Part model, mm, in its own coordinate system. Face numbers are marked on the shaded views. A direction names the side the tool comes from. Give positions to 0.01 mm unless a question says otherwise; leave off trailing zeros. Order: outer loops, then holes, each group sorted by start corner. A loop starts at its lowest first (then second) coordinate and runs counter-clockwise, first axis right, second up. Notation, with made-up numbers: (19, 33.5) - (46, 33.5) arc R17 ccw to (46, 40.5) - close; hole circle Ø3 at (62.5, 20.5). An arc over 180 degrees is marked (long way). One line per item, written item: value.
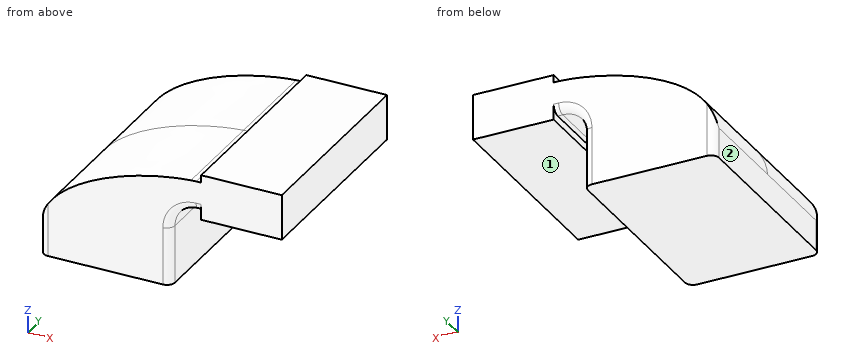
```python
from build123d import *

# Parameters (mm, degrees)
F0_W         = 25.4
F0_H         = 19.05
F0_H_2       = 4.7498
F0_H_3       = 4.7752
F1_DEPTH     = 65
F2_DEPTH     = 25.4
F3_DEPTH     = 7.9375
F5_T1_DEPTH  = 49.2252
F5_T3_DEPTH  = 53.34
F5_T5_DEPTH  = 3.175
F5_T8_ANGLE  = 90
F5_T10_ANGLE = 90


# Not quite as in the source:
# - a fillet or chamfer that OpenCascade refuses, or shapes differently, is made with other operations: its cross-section is extruded or revolved along the edge and cut away or added


with BuildPart() as f1:
    # F0 (on Front) → F1 (new body, symmetric)
    with BuildSketch(Plane.XZ):
        Polygon((22.225, 9.525), (-41.275, 9.525), (-41.275, -9.525), (41.275, -9.525), (41.275, 9.525), align=None)
        with BuildLine():
            add(Edge.make_bspline(
                [(-41.275, 9.525), (-39.5856284224, 39.4828766469), (13.870125209, 59.4306981306), (53.8854342407, 61.7722898912)],
                knots=[0, 0, 0, 0, 108.5245810491, 108.5245810491, 108.5245810491, 108.5245810491], degree=3))
            Line((-41.275, 9.525), (22.225, 9.525))
            Line((22.225, 9.525), (22.225, 27.0002))
            ThreePointArc((22.225, 27.0002), (31.3258777096, 50.5133948686), (53.8854342407, 61.7722898912))
        make_face()
        with BuildLine():
            Line((22.225, 27.0002), (22.225, 9.525))
            Line((22.225, 9.525), (41.275, 9.525))
            Line((41.275, 9.525), (41.275, 27.0002))
            ThreePointArc((41.275, 27.0002), (45.9246798487, 38.2255201513), (57.15, 42.8752))
            Line((57.15, 42.8752), (60.325, 42.8752))
            Line((60.325, 42.8752), (60.325, 61.9252))
            Line((60.325, 61.9252), (57.15, 61.9252))
            add(Edge.make_bspline(
                [(53.8854342407, 61.7722898912), (54.9842067368, 61.8365871986), (56.0728453275, 61.8876096574), (57.15, 61.9252)],
                knots=[108.5245810491, 108.5245810491, 108.5245810491, 108.5245810491, 111.5045361635, 111.5045361635, 111.5045361635, 111.5045361635], degree=3))
            ThreePointArc((53.8854342407, 61.7722898912), (31.3258777096, 50.5133948686), (22.225, 27.0002))
        make_face()
        with Locations((73.025, 52.4002)):
            Rectangle(F0_W, F0_H)
        with Locations((73.025, 64.3001)):
            Rectangle(F0_W, F0_H_2)
        with Locations((73.025, 40.4876)):
            Rectangle(F0_W, F0_H_3)
        Polygon((85.725, 66.675), (85.725, 61.9252), (85.725, 42.8752), (85.725, 38.1), (111.125, 38.1), (111.125, 66.675), align=None)
    extrude(amount=F1_DEPTH, both=True)

    # F0 (on Front) → F2 (join, symmetric)
    with BuildSketch(Plane.XZ):
        with BuildLine():
            Line((22.225, 27.0002), (22.225, 9.525))
            Line((22.225, 9.525), (41.275, 9.525))
            Line((41.275, 9.525), (41.275, 27.0002))
            ThreePointArc((41.275, 27.0002), (45.9246798487, 38.2255201513), (57.15, 42.8752))
            Line((57.15, 42.8752), (60.325, 42.8752))
            Line((60.325, 42.8752), (60.325, 61.9252))
            Line((60.325, 61.9252), (57.15, 61.9252))
            add(Edge.make_bspline(
                [(53.8854342407, 61.7722898912), (54.9842067368, 61.8365871986), (56.0728453275, 61.8876096574), (57.15, 61.9252)],
                knots=[108.5245810491, 108.5245810491, 108.5245810491, 108.5245810491, 111.5045361635, 111.5045361635, 111.5045361635, 111.5045361635], degree=3))
            ThreePointArc((53.8854342407, 61.7722898912), (31.3258777096, 50.5133948686), (22.225, 27.0002))
        make_face()
        with Locations((73.025, 52.4002)):
            Rectangle(F0_W, F0_H)
    extrude(amount=F2_DEPTH, both=True)

    # F0 (on Front) → F3 (join, symmetric)
    with BuildSketch(Plane.XZ):
        with BuildLine():
            add(Edge.make_bspline(
                [(-41.275, 9.525), (-39.5856284224, 39.4828766469), (13.870125209, 59.4306981306), (53.8854342407, 61.7722898912)],
                knots=[0, 0, 0, 0, 108.5245810491, 108.5245810491, 108.5245810491, 108.5245810491], degree=3))
            Line((-41.275, 9.525), (22.225, 9.525))
            Line((22.225, 9.525), (22.225, 27.0002))
            ThreePointArc((22.225, 27.0002), (31.3258777096, 50.5133948686), (53.8854342407, 61.7722898912))
        make_face()
    extrude(amount=F3_DEPTH, both=True)

    # F0 (on Front) → F4 (revolve)
    with BuildSketch(Plane.XZ):
        Polygon((85.725, 66.675), (85.725, 61.9252), (85.725, 42.8752), (85.725, 38.1), (111.125, 38.1), (111.125, 66.675), align=None)
    revolve(axis=Axis((85.725, 0, 52.3875), (0, 0, 1)))

    # F5: fillet of radius 5.08 on 8 edges, made by hand

    # F5_s2 → F5_t1 (cut)
    with BuildSketch(Plane.XY.offset(-22.225)):
        with BuildLine():
            ThreePointArc((41.275, -59.92), (39.7871024484, -63.5121024484), (36.195, -65))
            Line((36.195, -65), (41.275, -65))
            Line((41.275, -65), (41.275, -59.92))
        make_face()
        with BuildLine():
            ThreePointArc((41.275, 59.92), (39.7871024484, 63.5121024484), (36.195, 65))
            Line((36.195, 65), (41.275, 65))
            Line((41.275, 65), (41.275, 59.92))
        make_face()
    extrude(amount=F5_T1_DEPTH, mode=Mode.SUBTRACT)

    # F5_s4 → F5_t3 (cut)
    with BuildSketch(Plane.XY.offset(-22.225)):
        with BuildLine():
            ThreePointArc((-41.275, -59.92), (-39.7871024484, -63.5121024484), (-36.195, -65))
            Line((-36.195, -65), (-41.275, -65))
            Line((-41.275, -65), (-41.275, -59.92))
        make_face()
        with BuildLine():
            ThreePointArc((-41.275, 59.92), (-39.7871024484, 63.5121024484), (-36.195, 65))
            Line((-36.195, 65), (-41.275, 65))
            Line((-41.275, 65), (-41.275, 59.92))
        make_face()
    extrude(amount=F5_T3_DEPTH, mode=Mode.SUBTRACT)

    # F5_s6 → F5_t5 (cut)
    with BuildSketch(Plane.YZ.offset(57.15)):
        with BuildLine():
            ThreePointArc((59.92, 42.8752), (63.5121024484, 44.3630975516), (65, 47.9552))
            Line((65, 47.9552), (65, 42.8752))
            Line((65, 42.8752), (59.92, 42.8752))
        make_face()
        with BuildLine():
            ThreePointArc((-59.92, 42.8752), (-63.5121024484, 44.3630975516), (-65, 47.9552))
            Line((-65, 47.9552), (-65, 42.8752))
            Line((-65, 42.8752), (-59.92, 42.8752))
        make_face()
    extrude(amount=F5_T5_DEPTH, mode=Mode.SUBTRACT)

    # F5_s7 → F5_t8 (revolve, cut)
    with BuildSketch(Plane.XY.offset(27.0002)):
        with BuildLine():
            ThreePointArc((41.275, 59.92), (39.7871024484, 63.5121024484), (36.195, 65))
            Line((36.195, 65), (41.275, 65))
            Line((41.275, 65), (41.275, 59.92))
        make_face()
    revolve(axis=Axis((57.15, 65, 27.0002), (0, 1, 0)), revolution_arc=F5_T8_ANGLE, mode=Mode.SUBTRACT)

    # F5_s9 → F5_t10 (revolve, cut)
    with BuildSketch(Plane.XY.offset(27.0002)):
        with BuildLine():
            ThreePointArc((41.275, -59.92), (39.7871024484, -63.5121024484), (36.195, -65))
            Line((36.195, -65), (41.275, -65))
            Line((41.275, -65), (41.275, -59.92))
        make_face()
    revolve(axis=Axis((57.15, -65, 27.0002), (0, 1, 0)), revolution_arc=F5_T10_ANGLE, mode=Mode.SUBTRACT)


solid = f1.part
```
1) Pin check, flat tips, straight feed: pin 1 (1 mm diameter, centred on x = 14.5, y = 51.5, fed in from +Z); pin 2 (1.5 mm diameter, centred on y = 32.5, z = 35.5, fed in from +X); pin 3 (3.5 mm diameter, centred on x = 58.5, y = 16.5, fed in from -Z). Stop position of each tip, or through.
Outcome:
pin 1: stops at z = 54.82
pin 2: stops at x = 44.25
pin 3: stops at z = 42.87
2) Drill centre lines: line 1 along Z through (x, y) = (69, -31.5) (3 decimals); line 2 along X through (y, z) = (27, 3.5) (3 decimals); line 3 along X through (y, z) = (-29.5, 41) (3 decimals). Where is each one in solid material? Low to high. Write a range as from..to.
Outcome:
line 1: z = 38.1..66.675
line 2: x = -41.275..41.275
line 3: x = -17.262..49.665, 60.325..111.125
3) Which spindle directions (+Z, -Z, +X, -X, +Y, -Y) get a long thin tool onto all of the face, cutting with end or side? Do the marked faces 1 and 2. Say none if no direction does.
Outcome:
face 1: -Z, +X, +Y, -Y
face 2: +Z, -Z, -X, +Y, -Y
4) Cut at A-A, the plane x = 97. Give the cut face in (y, z) (3 decimals).
Outcome:
outline: (-65, 38.1) - (65, 38.1) - (65, 66.675) - (-65, 66.675) - close
